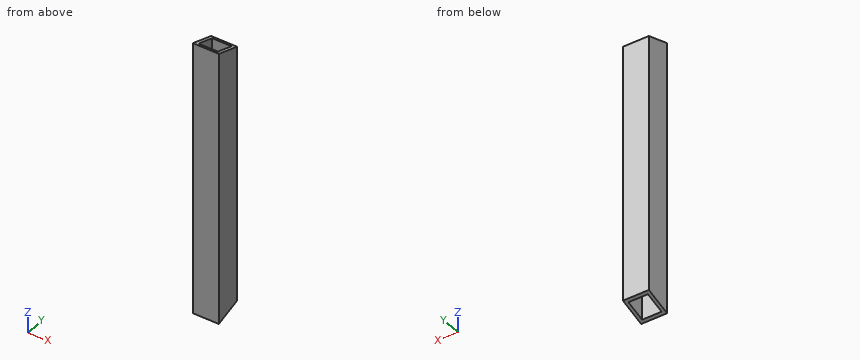
Autodesk Inventor part; units mm, degrees
ref_plane "YZ Plane" through (0, 0, 0) normal (1, 0, 0) x (0, 1, 0)
ref_plane "XZ Plane" through (0, 0, 0) normal (0, 1, 0) x (-1, 0, 0)
ref_plane "XY Plane" through (0, 0, 0) normal (0, 0, 1) x (1, 0, 0)
sketch "Sketch1" plane through (0, 0, 0) normal (0, 0, 1) x (1, 0, 0)
  line L0 (0, 0) -> (25.4, 0)
  line L1 (25.4, 0) -> (25.4, 25.4)
  line L2 (25.4, 25.4) -> (0, 25.4)
  line L3 (0, 25.4) -> (0, 0)
  line L4 (0, 0) -> (0, 3.175)
  line L5 (0, 3.175) -> (3.175, 3.175)
  line L6 (3.175, 3.175) -> (22.225, 3.175)
  line L7 (22.225, 3.175) -> (22.225, 22.225)
  line L8 (22.225, 22.225) -> (3.175, 22.225)
  line L9 (3.175, 22.225) -> (3.175, 3.175)
  dimension "d0" = 25.4
  dimension "d1" = 25.4
  dimension "d2" = 3.175
  dimension "d3" = 3.175
  dimension "d4" = 19.05
  dimension "d5" = 19.05
extrude "Extrusion1" add sketch "Sketch1" along normal blind 267.462
sketch "Sketch2" plane through (25.4, 0, 0) normal (1, 0, 0) x (0, 0, -1)
  line L0 (0, 0) -> (0, 25.4)
  line L1 (0, 25.4) -> (-267.462, 25.4)
  line L2 (-267.462, 0) -> (-267.462, 25.4)
  line L3 (-267.462, 0) -> (-259.4388, 25.4)
  line L4 (-267.462, 0) -> (-240.825, 0) construction
  line L5 (0, 0) -> (-8.0232, 25.4)
  line L6 (0, 0) -> (26.637, 0) construction
  line L7 (-259.4388, 25.4) -> (-267.462, 25.4)
  line L8 (-267.462, 0) -> (-267.462, 25.4)
  line L9 (-8.0232, 25.4) -> (0, 25.4)
  line L10 (0, 25.4) -> (0, 0)
  dimension "d8" = 72.47
  dimension "d9" = 107.53
extrude "Extrusion2" cut sketch "Sketch2" against normal up to next
properties part number "midBrace"
Can you work these out from the model? Positions are in its coordinate system, mm. Give positions to 0.01 mm unless a question says otherwise; leave off trailing zeros. Write each loop counter-clockwise with the first axis right and the second up, starting at its lowest first coordinate (ties: lowest second). Pieces come first, ordered by that corner, then holes. Notation, with made-up numbers: M 63,-2.75 L 119,-2.75 A15 cw 119,10.25 Z; hole C 65,47.25 d5. An arc over 180 degrees is marked long. Answer in a Markdown table with one row per item. Add a question column.
Item 1: Please list where these lines run through material, in increasing order: L1, parallel to X at y = 21.25, z = 165 (3 decimals); L2, parallel to Z at x = 1, y = 16.75.
Item 2: Imagine slicing it at A-A, the plane z = 23. Write out the boundary of the cut face in (x, y) (3 decimals), plus the area to 3 significant figures.
Item 3: Imagine slicing it at C-C, the plane y = 7.75. Write out the boundary of the cut face in (x, z) (3 decimals), plus the area to 3 significant figures.
Item 4: For pin 1 Ø12 at (x, y) = (13.5, 11) entering from -Z, with a flat end and sliding along its axis, tell me the tip position at first contact or that it passes through.
Item 5: Imagine slicing it at B-B, the plane x = 17. Write out the boundary of the cut face in (y, z) (3 decimals), plus the area to 3 significant figures.
Evaluation:
| question | item | result |
|---|---|---|
| 1 | L1 | x = 0 to 3.175, 22.225 to 25.4 |
| 1 | L2 | z = 5.29 to 262.17 |
| 2 | outline | M 0,0 L 25.4,0 L 25.4,25.4 L 0,25.4 Z; hole M 3.175,3.175 L 22.225,3.175 L 22.225,22.225 L 3.175,22.225 Z |
| 2 | area | 282 mm² |
| 3 | outline | M 0,2.448 L 3.175,2.448 L 3.175,265.014 L 0,265.014 Z; M 22.225,2.448 L 25.4,2.448 L 25.4,265.014 L 22.225,265.014 Z |
| 3 | area | 1,670 mm² |
| 4 | pin 1 | passes through |
| 5 | outline | M 0,0 L 3.175,1.003 L 3.175,266.459 L 0,267.462 Z; M 22.225,7.02 L 25.4,8.023 L 25.4,259.439 L 22.225,260.442 Z |
| 5 | area | 1,650 mm² |
